Verification items for the finished model (mm, model axes). Face numbers are marked on the shaded views. A direction names the side the tool comes from. Give positions to 0.01 mm unless a question says otherwise; leave off trailing zeros. Write each loop counter-clockwise with the first axis right and the second up, starting at its lowest first coordinate (ties: lowest second). Pieces come first, ordered by that corner, then holes. Notation, with made-up numbers: (75, 47) - (107, 47) arc R26 cw to (107, 81) - close; hole circle Ø6 at (29.25, 42). An arc over 180 degrees is marked (long way). Put each result on its own line as item: value.
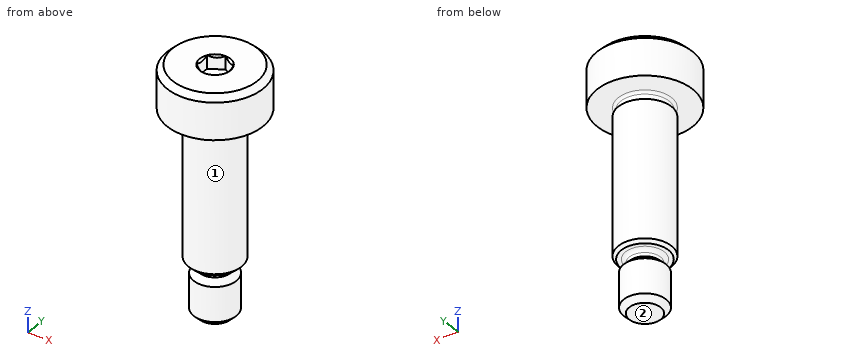
from build123d import *

# Parameters (mm, degrees)
CUT_EXTRUDE1_DEPTH = 1.25
SKETCH4_R          = 1.443375673
CUT_EXTRUDE2_DEPTH = 1.25
CUT_EXTRUDE2_DRAFT = -45


with BuildPart() as part:
    # Sketch2 → Revolve1 (revolve)
    with BuildSketch(Plane(origin=(0, 0, 0), x_dir=(0, 0, -1), z_dir=(1, 0, 0)), mode=Mode.PRIVATE) as revolve1_sk:
        with BuildLine():
            Line((11.5, 0), (11.5, 1.475))
            Line((11.5, 1.475), (10.975, 2))
            Line((10.975, 2), (7.73044056, 2))
            Line((7.73044056, 2), (7.2, 1.46955944))
            Line((7.2, 1.46955944), (6.85, 1.46955944))
            ThreePointArc((6.85, 1.46955944), (6.602512627, 1.572072067), (6.5, 1.81955944))
            Line((6.5, 1.81955944), (6.5, 2.22))
            Line((6.5, 2.22), (6.22, 2.5))
            Line((6.22, 2.5), (-6.665284937, 2.5))
            Line((-6.665284937, 2.5), (-6.8, 2.266666667))
            Line((-6.8, 2.266666667), (-7.266666667, 2.266666667))
            ThreePointArc((-7.266666667, 2.266666667), (-7.431658249, 2.335008418), (-7.5, 2.5))
            Line((-7.5, 2.5), (-7.5, 4.5))
            Line((-7.5, 4.5), (-10.975, 4.5))
            Line((-10.975, 4.5), (-11.5, 3.975))
            Line((-11.5, 3.975), (-11.5, 0))
            Line((-11.5, 0), (11.5, 0))
        make_face()
    revolve(revolve1_sk.sketch.rotate(Axis((0, 0, 11.5), (0, 0, -1)), 180), axis=Axis((0, 0, 11.5), (0, 0, -1)))

    # Sketch3 → Cut-Extrude1 (cut)
    with BuildSketch(Plane.XY.offset(11.5)):
        Polygon((0, 1.443375673), (-1.25, 0.721687836), (-1.25, -0.721687836), (0, -1.443375673), (1.25, -0.721687836), (1.25, 0.721687836), align=None)
    extrude(amount=-CUT_EXTRUDE1_DEPTH, mode=Mode.SUBTRACT)


with BuildPart() as cut_extrude2_tool:
    # Sketch4 → Cut-Extrude2 (with draft: the straight prism first)
    with BuildSketch(Plane.XY.offset(11.5)):
        Circle(SKETCH4_R)
    extrude(amount=-CUT_EXTRUDE2_DEPTH)
    # Cut-Extrude2: the draft: its side faces are tilted about the plane it starts from
    cut_extrude2_sides = [cut_extrude2_tool.faces().sort_by_distance(p)[0] for p in [
        (-1.443375673, 0, 10.875),
    ]]
    draft(cut_extrude2_sides, Plane.XY.offset(11.5), CUT_EXTRUDE2_DRAFT)


with BuildPart() as part_1:
    add(part.part)

    # Cut-Extrude2: cut by cut_extrude2_tool
    add(cut_extrude2_tool.part, mode=Mode.SUBTRACT)


solid = part_1.part
Q1. Section check B-B, the plane z = 9.5. Record the cut outline in (x, y), plus the area to 3 significant figures.
Answers follow:
outline: circle Ø9 at (0, 0)
area: 63.6 mm2
Q2. Section check A-A, the plane z = -4.5. Record the cut outline in (x, y), plus the area to 3 significant figures.
Answers follow:
outline: circle Ø5 at (0, 0)
area: 19.6 mm2
Q3. Set-up check for the marked faces 1 and 2: record each of +Z, -Z, +X, -X, +Y, -Y from which the full face is reachable in a straight line by a thin tool's end or side.
Answers follow:
face 1: -Z
face 2: -Z, +X, -X, +Y, -Y
Q4. Go/stop test with flat-tipped pins: pin 1 Ø3 at (x, z) = (-3, -5.5) entering from +Y; pin 2 Ø1.5 at (y, z) = (0.5, 0) entering from -X; pin 3 Ø5 at (x, z) = (-2, -1) entering from -Y. Record where each tip stops, or that it passes through.
Answers follow:
pin 1: stops at y = 2
pin 2: stops at x = -2.5
pin 3: stops at y = -2.5
Q5. Scan lines: line 1 along Z through (x, y) = (2.5, 1.25); line 2 along Z through (x, y) = (0.75, 0.5); line 3 along Y through (x, z) = (1.5, 5.25). Record each from-to range of solid material in increasing order.
Answers follow:
line 1: z = 7.5 to 11.5
line 2: z = -11.5 to 10.25
line 3: y = -2 to 2
